```python
from build123d import *

# Parameters (mm, degrees)
SKETCH1_W           = 50
SKETCH1_H           = 50
BOSS_EXTRUDE1_DEPTH = 50
SKETCH2_W           = 45
SKETCH2_H           = 45
CUT_EXTRUDE1_DEPTH  = 45
FILLET2_SIZE        = 5
FILLET3_SIZE        = 3


with BuildPart() as part:
    # Sketch1 → Boss-Extrude1 (new body)
    with BuildSketch(Plane(origin=(0, 0, 0), x_dir=(1, 0, 0), z_dir=(0, 1, 0))):
        Rectangle(SKETCH1_W, SKETCH1_H)
    extrude(amount=BOSS_EXTRUDE1_DEPTH)

    # Sketch2 → Cut-Extrude1 (cut)
    with BuildSketch(Plane(origin=(0, 50, 0), x_dir=(1, 0, 0), z_dir=(0, 1, 0))):
        Rectangle(SKETCH2_W, SKETCH2_H)
    extrude(amount=-CUT_EXTRUDE1_DEPTH, mode=Mode.SUBTRACT)

    # Fillet2
    fillet2_edges = [part.edges().sort_by_distance(p)[0] for p in [
        (0, 0, 25),
        (-25, 0, 0),
        (0, 0, -25),
        (25, 0, 0),
        (25, 25, 25),
        (-25, 25, 25),
        (-25, 25, -25),
        (25, 25, -25),
    ]]
    chamfer(fillet2_edges, length=FILLET2_SIZE - 0.0001)  # a hair under: the kernel refuses the full size

    # Fillet3
    fillet3_edges = [part.edges().sort_by_distance(p)[0] for p in [
        (-22.5, 27.5, -22.5),
        (-22.5, 27.5, 22.5),
        (22.5, 27.5, 22.5),
        (22.5, 27.5, -22.5),
    ]]
    chamfer(fillet3_edges, length=FILLET3_SIZE)


solid = part.part
```
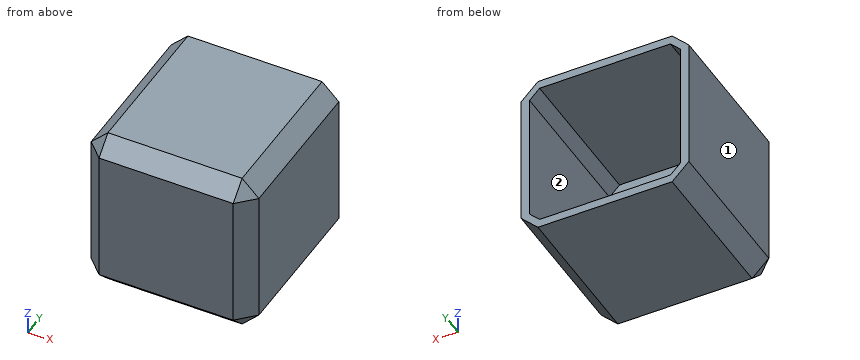
Model file for the job. Use its own axes, mm. Face numbers are marked on the shaded views. A direction names the side the tool comes from. Coordinates: 2 decimals unless noted, no trailing zeros. Order: outer loops, then holes, each group sorted by start corner. A loop starts at its lowest first (then second) coordinate and runs counter-clockwise, first axis right, second up. Notation, with made-up numbers: M 7.5,16.5 L 55.5,16.5 A17 ccw 55.5,43.5 Z; hole C 76.5,9 d6. An arc over 180 degrees is marked long. Answer as CSV lines item,"result".
(1) Band-saw the part on B-B, the plane z = 4. List the corners of the cut face in (x, y).
Geometry says:
outline,"M -25,5 L -20,0 L 20,0 L 25,5 L 25,50 L 22.5,50 L 22.5,5 L -22.5,5 L -22.5,50 L -25,50 Z"
(2) 3-axis set-ups, long thin cutter, end or side, ignore diameter. For the marked faces 1 and 2: which of +Z, -Z, +X, -X, +Y, -Y reach the whole face in a straight line?
Geometry says:
face 1,"+Z, -Z, -X, +Y, -Y"
face 2,"+Y"
(3) Band-saw the part on A-A, the plane y = 16.5. List the corners of the cut face in (x, z), then the cut area to 3 significant figures.
Geometry says:
outline,"M -25,-20 L -20,-25 L 20,-25 L 25,-20 L 25,20 L 20,25 L -20,25 L -25,20 Z; hole M -22.5,-19.5 L -19.5,-22.5 L 19.5,-22.5 L 22.5,-19.5 L 22.5,19.5 L 19.5,22.5 L -19.5,22.5 L -22.5,19.5 Z"
area,"443 mm2"
(4) Flat gauge pin, fed straight in: pin 1 (2 mm diameter, centred on x = -1.5, z = 11, fed in from +Y). Where does the tip first touch, or does it go through?
Geometry says:
pin 1,"stops at y = 5"
(5) Band-saw the part on C-C, the plane x = 17. List the corners of the cut face in (y, z), then the cut area to 3 significant figures.
Geometry says:
outline,"M 0,-20 L 5,-25 L 50,-25 L 50,-22.5 L 5,-22.5 L 5,22.5 L 50,22.5 L 50,25 L 5,25 L 0,20 Z"
area,"450 mm2"
(6) Wall check: line 1 along Z through (x, y) = (16, 19); line 2 along Y through (x, z) = (-10, -9.5). Give the ranges that are in metal, low to high.
Geometry says:
line 1,"z = -25 to -22.5, 22.5 to 25"
line 2,"y = 0 to 5"
